The listing builds one solid part. Answer for the finished solid, in the listing's coordinates (mm). A direction names the side the tool comes from. Give positions to 0.01 mm unless a question says otherwise; leave off trailing zeros. Loops run counter-clockwise (first coordinate to the right, second up) from the corner with the lowest first, then second, coordinate; pieces in that order, holes last. Notation, with made-up numbers: M -16,-4.5 L 22,-4.5 A25 ccw 22,10.5 Z; hole C 73,17.25 d7. An arc over 180 degrees is marked long. Return JSON: item names as keys, results as strings.
from build123d import *

# Parameters (mm, degrees)
SKETCH1_W            = 95
SKETCH1_H            = 95
BOSS_EXTRUDE1_DEPTH  = 10
FILLET1_R            = 10
BOSS_EXTRUDE2_DEPTH  = 3
SKETCH5_W            = 4.733468523
SKETCH5_H            = 15.739624206
SKETCH5_W_2          = 4.285968544
SKETCH5_W_3          = 4.922499766
CUT_EXTRUDE1_DEPTH   = 10
SKETCH14_W           = 21
SKETCH14_H           = 9
CUT_EXTRUDE2_DEPTH   = 10
SKETCH16_W           = 21.335954762
SKETCH16_H           = 13.618694529
BOSS_EXTRUDE7_DEPTH  = 10
SKETCH20_W           = 21
SKETCH20_H           = 1.5
BOSS_EXTRUDE13_DEPTH = 20


with BuildPart() as part:
    # Sketch1 → Boss-Extrude1 (new body)
    with BuildSketch(Plane(origin=(-45.242822535, 0, -5.598622024), x_dir=(1, 0, 0), z_dir=(0, 1, 0))):
        Rectangle(SKETCH1_W, SKETCH1_H)
    extrude(amount=BOSS_EXTRUDE1_DEPTH)

    # Fillet1
    fillet1_edges = [part.edges().sort_by_distance(p)[0] for p in [
        (2.257177465, 5, 41.901377976),
        (-92.742822535, 5, 41.901377976),
        (-92.742822535, 5, -53.098622024),
        (2.257177465, 5, -53.098622024),
    ]]
    fillet(fillet1_edges, radius=FILLET1_R)

    # Sketch4 → Boss-Extrude2 (add)
    with BuildSketch(Plane(origin=(-45.242822535, 0, -5.598622024), x_dir=(1, 0, 0), z_dir=(0, -1, 0))):
        with BuildLine():
            Line((-46, 37.5), (-46, -37.5))
            ThreePointArc((-46, -37.5), (-43.51040764, -43.51040764), (-37.5, -46))
            Line((-37.5, -46), (37.5, -46))
            ThreePointArc((37.5, -46), (43.51040764, -43.51040764), (46, -37.5))
            Line((46, -37.5), (46, 37.5))
            ThreePointArc((46, 37.5), (43.51040764, 43.51040764), (37.5, 46))
            Line((37.5, 46), (-37.5, 46))
            ThreePointArc((-37.5, 46), (-43.51040764, 43.51040764), (-46, 37.5))
        make_face()
    extrude(amount=BOSS_EXTRUDE2_DEPTH)

    # Sketch5 → Cut-Extrude1 (cut)
    with BuildSketch(Plane(origin=(-45.242822535, 10, -5.598622024), x_dir=(1, 0, 0), z_dir=(0, 1, 0))):
        with Locations((-36.445515764, -32.326942183)):
            Rectangle(SKETCH5_W, SKETCH5_H)
        with Locations((-30.082156711, -32.326942183)):
            Rectangle(SKETCH5_W_2, SKETCH5_H)
        with Locations((-23.365813302, -32.326942183)):
            Rectangle(SKETCH5_W_3, SKETCH5_H)
    extrude(amount=-CUT_EXTRUDE1_DEPTH, mode=Mode.SUBTRACT)

    # Sketch14 → Cut-Extrude2 (cut)
    with BuildSketch(Plane(origin=(0, 10, 0), x_dir=(1, 0, 0), z_dir=(0, 1, 0))):
        with Locations((-75.521903194, -8.192829138)):
            Rectangle(SKETCH14_W, SKETCH14_H)
    extrude(amount=-CUT_EXTRUDE2_DEPTH, mode=Mode.SUBTRACT)

    # Sketch16 → Boss-Extrude7 (add)
    with BuildSketch(Plane(origin=(0, 0, 0), x_dir=(1, 0, 0), z_dir=(0, 1, 0))):
        with Locations((-75.859791542, 2.420926633)):
            Rectangle(SKETCH16_W, SKETCH16_H)
    extrude(amount=BOSS_EXTRUDE7_DEPTH)

    # Sketch20 → Boss-Extrude13 (add)
    with BuildSketch(Plane(origin=(0, 10, 0), x_dir=(1, 0, 0), z_dir=(0, 1, 0))):
        with Locations((-75.800790681, -4.586951107)):
            Rectangle(SKETCH20_W, SKETCH20_H)
    extrude(amount=BOSS_EXTRUDE13_DEPTH)


solid = part.part
(1) Straight lines are drawn through the part: line 1 along Z through (x, y) = (-76, 6); line 2 along Y through (x, z) = (-34.5, -42.5); line 3 along Z through (x, y) = (-67.5, 26). For each, find the intervals that lie inside material, in ascending order.
Values follow:
{"line 1": "-53.1 to 4.39, 12.69 to 18.86, 34.6 to 41.9", "line 2": "-3 to 10", "line 3": "3.84 to 5.34"}
(2) The part is cut by section D-D (z = 36.5). Determine the outline of the cut face in (x, y), and give its area (3 significant figures).
Values follow:
{"outline": "M -91.62,0 L -89.89,0 L -89.89,-3 L -0.59,-3 L -0.59,0 L 1.14,0 L 1.14,10 L -91.62,10 Z", "area": "1,200 mm²"}
(3) The part is cut by section B-B (x = -81). Determine the outline of the cut face in (y, z), and give its area (3 significant figures).
Values follow:
{"outline": "M -3,-51.6 L 0,-51.6 L 0,-53.1 L 10,-53.1 L 10,3.84 L 30,3.84 L 30,5.34 L 10,5.34 L 10,4.39 L 0,4.39 L 0,12.69 L 10,12.69 L 10,18.86 L 0,18.86 L 0,34.6 L 10,34.6 L 10,41.9 L 0,41.9 L 0,40.4 L -3,40.4 Z", "area": "1,020 mm²"}
(4) Determine the mould class of faces 4 (the flat face through (-82, 5, 18.859)), 5 (the cylindrical face through (-88.687, -1.479, 37.978)), 6 (the flat face through (-46, 10, -6)) for opening direction X: released by +X, released by -X, zero draft, split by the parting line, or undercut.
Values follow:
{"face 4": "undercut", "face 5": "released by -X", "face 6": "zero draft"}
(5) A tool of negligible diameter and unlimited length cuts with its end or side. For faces 1 (the flat face through (-82, 5, 34.598)), 2 (the flat face through (-84, 0, -52)), 3 (the flat face through (-76, 20, 5.337)), from which of +Z, -Z, +X, -X, +Y, -Y can it reach the whole face along a straight path? Write none if from no direction.
Values follow:
{"face 1": "+Y", "face 2": "-Y", "face 3": "+Z, +X, -X, +Y"}
(6) Given pin 1 (4 mm diameter, centred on x = -80.5, z = 26.5, fed in from +Y); pin 2 (1.2 mm diameter, centred on y = 18.5, z = 4.5, fed in from -X); pin 3 (1.6 mm diameter, centred on y = 17, z = 4.5, fed in from +X), each flat-ended and moving along its own axis, determine where each tip first touches the part or whether it passes through.
Values follow:
{"pin 1": "y = 10", "pin 2": "x = -86.3", "pin 3": "x = -65.3"}
(7) The part is cut by section A-A (z = 8.5). Determine the outline of the cut face in (x, y), and give its area (3 significant figures).
Values follow:
{"outline": "M -92.74,0 L -91.24,0 L -91.24,-3 L 0.76,-3 L 0.76,0 L 2.26,0 L 2.26,10 L -65.02,10 L -65.02,0 L -86.02,0 L -86.02,10 L -92.74,10 Z", "area": "1,020 mm²"}
(8) The part is cut by section C-C (y = 18.5). Determine the outline of the cut face in (x, z).
Values follow:
{"outline": "M -86.3,3.84 L -65.3,3.84 L -65.3,5.34 L -86.3,5.34 Z"}
